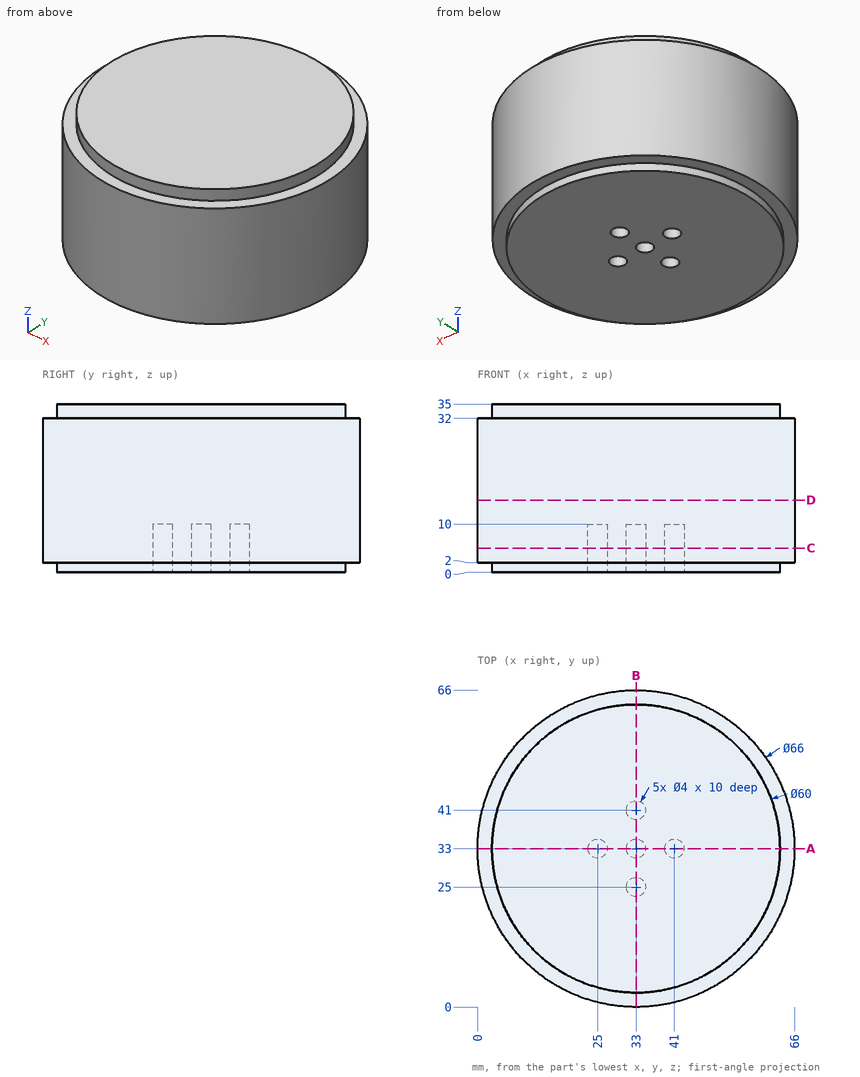
Design review of the part shown in the three views and the two pictorial views. Dimensions are in mm from the part's minimum x, y and z. Give positions to 0.01 mm unless a question says otherwise; leave off trailing zeros. Loops run counter-clockwise (first coordinate to the right, second up) from the corner with the lowest first, then second, coordinate; pieces in that order, holes last. Notation, with made-up numbers: M 20,80 L 41,80 A32 ccw 41,113 Z; hole C -3.75,52.25 d8. An arc over 180 degrees is marked long. Put each result on its own line as item: value. Start each with the question number.
(1) Wall thickness on L1, parallel to Y at x = 32.5, z = 5; L2, parallel to Z at x = 59, y = 50; L3, parallel to Y at x = 41, z = 6: over which ranges is each line inside the solid? List them lowest first.
(2) For pin 1 (5 mm diameter, centred on y = 34, z = 22.5, fed in from +X); pin 2 (1 mm diameter, centred on y = 38.5, z = 29.5, fed in from +X); pin 3 (4 mm diameter, centred on x = 7.5, z = 4.5, fed in from +Y); pin 4 (2.5 mm diameter, centred on x = 33, y = 25, fed in from -Z), all flat-tipped, find the tip position at first contact; note any pin that passes through.
(3) Add section C-C, the plane z = 5. Write out the cut boundary in (x, y), then the cut area to 3 significant figures.
(4) Add section A-A, the plane y = 33. Write out the cut boundary in (x, z).
(5) Add section D-D, the plane z = 15. Write out the cut boundary in (x, y).
Result:
1. L1: y = 0 to 23.06, 26.94 to 31.06, 34.94 to 39.06, 42.94 to 66
1. L2: z = 2 to 32
1. L3: y = 0.98 to 31, 35 to 65.02
2. pin 1: stops at x = 66
2. pin 2: stops at x = 65.62
2. pin 3: stops at y = 56.17
2. pin 4: stops at z = 10
3. outline: C 33,33 d66; hole C 25,33 d4; hole C 33,25 d4; hole C 33,33 d4; hole C 33,41 d4; hole C 41,33 d4
3. area: 3,360 mm^2
4. outline: M 0,2 L 3,2 L 3,0 L 23,0 L 23,10 L 27,10 L 27,0 L 31,0 L 31,10 L 35,10 L 35,0 L 39,0 L 39,10 L 43,10 L 43,0 L 63,0 L 63,2 L 66,2 L 66,32 L 63,32 L 63,35 L 3,35 L 3,32 L 0,32 Z
5. outline: C 33,33 d66
